Solid Edge part; units mm, degrees
sketch "Sketch1" plane through (0, 0, 0) normal (0, -1, 0) x (1, 0, 0)
  line L0 (-10.1036, 17.5) -> (-20.2073, 0)
  line L1 (-20.2073, 0) -> (-10.1036, -17.5)
  line L2 (-10.1036, -17.5) -> (10.1036, -17.5)
  line L3 (10.1036, -17.5) -> (20.2073, 0)
  line L4 (20.2073, 0) -> (10.1036, 17.5)
  line L5 (10.1036, 17.5) -> (-10.1036, 17.5)
extrude "Protrusion1" add sketch "Sketch1" against normal blind 15
sketch "Sketch2" plane through (0, 0, 0) normal (0, -1, 0) x (1, 0, 0)
  circle A0 centre (0, 0) radius 11
extrude "ExtrudedCutout_1" cut sketch "Sketch2" against normal blind 49.2939
cosmetic_thread "Thread1"
Here's how the part is built. I have some questions about the finished solid (model axes, mm). Give positions to 0.01 mm unless a question says otherwise; leave off trailing zeros. Order: outer loops, then holes, each group sorted by start corner. A loop starts at its lowest first (then second) coordinate and runs counter-clockwise, first axis right, second up. Notation, with made-up numbers: M -28.5,5.25 L -10.5,5.25 A27 cw -10.5,39.25 Z; hole C 54.25,11.5 d9. An arc over 180 degrees is marked long. Use a Markdown table: item, result. Add a question column.
1. Suppose I cut it at D-D (x = 15). List the corners of the cut face in (y, z) for me.
2. Suppose I cut it at B-B (y = 4). List the corners of the cut face in (x, z) for me.
3. Suppose I cut it at C-C (z = -1.5). List the corners of the cut face in (x, y) for me, and give its area (3 significant figures).
4. Suppose I cut it at A-A (x = 0). List the corners of the cut face in (y, z) for me.
5. If we mould it in two halves opening along X, with no side actions, what happens to faces 1 (the flat face through (15.085, 7.395, -8.872)), 2 (the cylindrical face through (-2.38, 7.4, -10.74)), 3 (the flat face through (0, 7, 17.5))? For each: +X half, -X half, draft (parallel to the pull), parting line (faces both ways), or undercut.
6. I need wall thicknesses on probe 1 along Z at (x, y) = (0, 10.5); probe 2 along X at (y, z) = (10, -6.5); probe 3 along Z at (x, y) = (-9, 5). Which ranges of each line are inside material? Lowest first, please. Write a range as from..to.
7. For pin 1 Ø6 at (y, z) = (13.5, -5) entering from -X; pin 2 Ø8 at (y, z) = (7.5, 14) entering from -X, each with a flat end and sliding along its axis, tell me the tip position at first contact or that it passes through.
Results list:
| question | item | result |
|---|---|---|
| 1 | outline | M 0,-9.02 L 15,-9.02 L 15,9.02 L 0,9.02 Z |
| 2 | outline | M -20.21,0 L -10.1,-17.5 L 10.1,-17.5 L 20.21,0 L 10.1,17.5 L -10.1,17.5 Z; hole C 0,0 d22 |
| 3 | outline | M -19.34,0 L -10.9,0 L -10.9,15 L -19.34,15 Z; M 10.9,0 L 19.34,0 L 19.34,15 L 10.9,15 Z |
| 3 | area | 253 mm² |
| 4 | outline | M 0,-17.5 L 15,-17.5 L 15,-11 L 0,-11 Z; M 0,11 L 15,11 L 15,17.5 L 0,17.5 Z |
| 5 | face 1 | +X half |
| 5 | face 2 | undercut |
| 5 | face 3 | draft |
| 6 | probe 1 | z = -17.5..-11, 11..17.5 |
| 6 | probe 2 | x = -16.45..-8.87, 8.87..16.45 |
| 6 | probe 3 | z = -17.5..-6.32, 6.32..17.5 |
| 7 | pin 1 | stops at x = -19.05 |
| 7 | pin 2 | stops at x = -14.43 |
